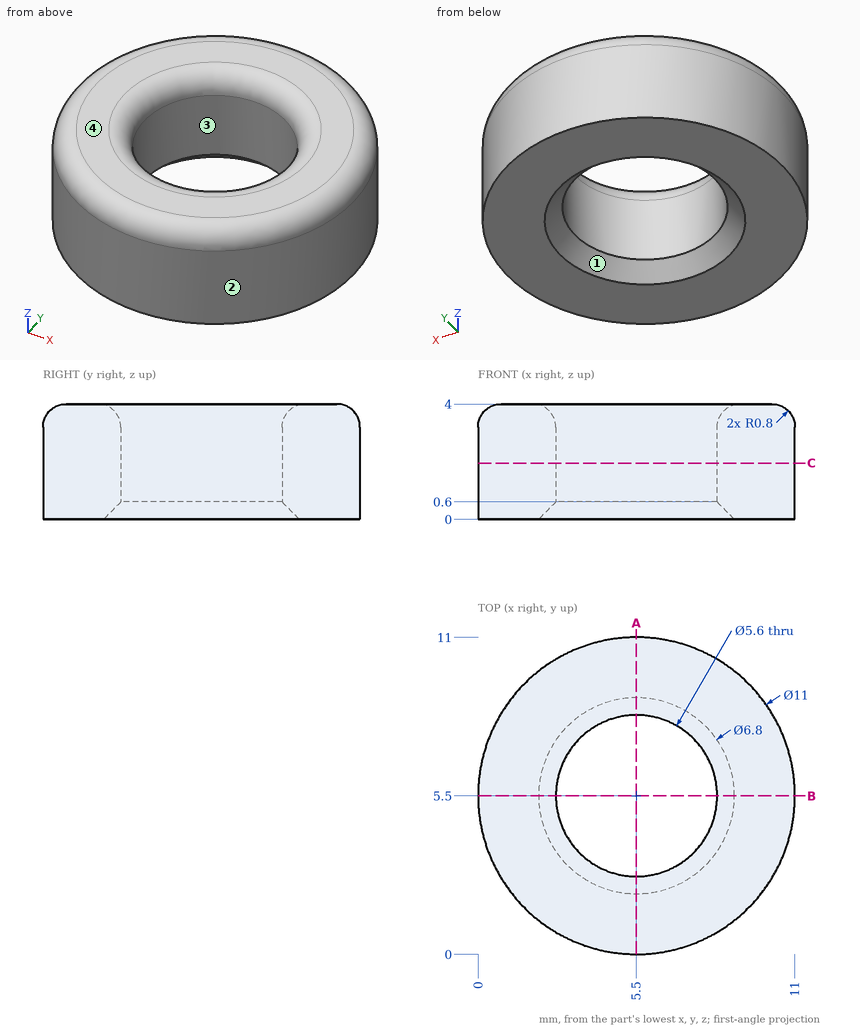
Geometry check sheet. Reference: drawing and pictorial views, mm from the part's lowest x, y, z. Coordinates: 2 decimals unless noted, no trailing zeros. Order: outer loops, then holes, each group sorted by start corner. A loop starts at its lowest first (then second) coordinate and runs counter-clockwise, first axis right, second up.
Item 1: Section check C-C (z = 1.95). Enter the section's corners in (x, y).
Item 2: Mould release check, pull along X, two halves, no side actions. Record for the marked faces 1, 2, 3 and 4: released by +X, released by -X, zero draft, split by the parting line, or undercut.
Item 3: Section check A-A (x = 5.5). Enter the section's corners in (y, z).
Item 4: Depth check by flat-ended pin: pin 1 (1 mm diameter, centred on x = 7.5, z = 3, fed in from +Y); pin 2 (2 mm diameter, centred on y = 2, z = 0.5, fed in from -X). Enter the tip coordinate at first touch or a pass-through.
Item 5: Scan lines: line 1 along Y through (x, z) = (5.5, 1.7); line 2 along X through (y, z) = (3.25, 1.6); line 3 along Y through (x, z) = (6.25, 3.6). Record each from-to range of solid material in increasing order.
Check sheet entries:
1. outline: circle Ø11 at (5.5, 5.5); hole circle Ø5.6 at (5.5, 5.5)
2. face 1: undercut
2. face 2: split by the parting line
2. face 3: undercut
2. face 4: zero draft
3. outline: (0, 0) - (2.1, 0) - (2.7, 0.6) - (2.7, 3.2) arc R0.8 ccw to (1.9, 4) - (0.8, 4) arc R0.8 ccw to (0, 3.2) - close; (8.3, 0.6) - (8.9, 0) - (11, 0) - (11, 3.2) arc R0.8 ccw to (10.2, 4) - (9.1, 4) arc R0.8 ccw to (8.3, 3.2) - close
4. pin 1: stops at y = 10.79
4. pin 2: stops at x = 0.6
5. line 1: y = 0 to 2.7, 8.3 to 11
5. line 2: x = 0.48 to 3.83, 7.17 to 10.52
5. line 3: y = 0.16 to 2.69, 8.31 to 10.84
